Check sheet for the modelled part. Datum: model origin and axes. Units: mm. Face numbers are marked on the shaded views. Give positions to 0.01 mm unless a question says otherwise; leave off trailing zeros. Write each loop counter-clockwise with the first axis right and the second up, starting at its lowest first coordinate (ties: lowest second). Pieces come first, ordered by that corner, then holes. Notation, with made-up numbers: M 2.25,26.25 L 57.25,26.25 A15 cw 57.25,38.25 Z; hole C 89,89 d2. An arc over 180 degrees is marked long. Use CSV: the item, a comma, the result in double quotes. Start each with the question number.
1. Scan lines: line 1 (Y direction, x = 0, z = 7); line 2 (Z direction, x = 18.5, y = 7); line 3 (Z direction, x = 4, y = -2). Record each from-to range of solid material in increasing order.
2. Cross-section at B-B, the plane y = 38.5. Enter the section's corners in (x, z).
3. Mould release check, pull along X, two halves, no side actions. Record for the marked faces 1, 2 and 3: +X half, -X half, draft (parallel to the pull), parting line (faces both ways), or undercut.
4. Cross-section at C-C, the plane z = 6.5. Enter the section's corners in (x, y), and give its area (3 significant figures).
5. Depth check by flat-ended pin: P1, Ø3, axis at y = -1, z = 20.5, coming from the +X side; P2, Ø8, axis at x = -7, y = 43.5, coming from the -Z side; P3, Ø10, axis at x = -52, z = 5, coming from the +Y side; P4, Ø2, axis at x = 9.5, z = 28, coming from the -Y side. Enter the tip coordinate at first touch or a pass-through.
6. Cross-section at A-A, the plane x = 52. Enter the section's corners in (y, z).
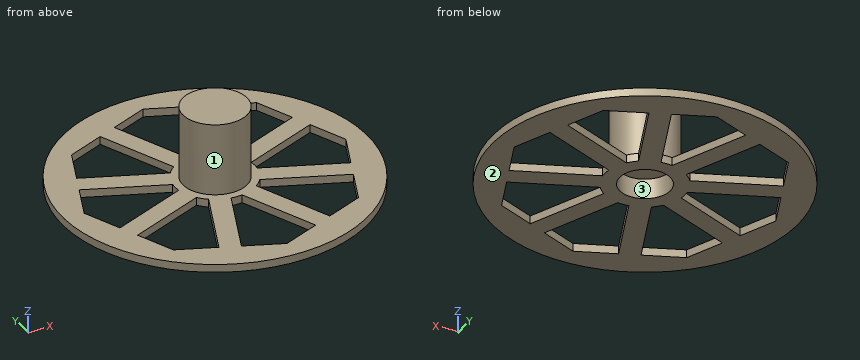
from build123d import *

# Parameters (mm, degrees)
F0_R     = 16
F1_DEPTH = 40
F2_R     = 12.6
F3_DEPTH = 10
F4_R     = 76
F4_R_2   = 16
F5_DEPTH = 4
F7_DEPTH = 4


with BuildPart() as f1:
    # F0 (on Top) → F1 (new body)
    with BuildSketch(Plane.XY):
        Circle(F0_R)
    extrude(amount=F1_DEPTH)

    # F2 (on face) → F3 (cut)
    with BuildSketch(Plane(origin=(0, 0, 0), x_dir=(1, 0, 0), z_dir=(0, 0, -1))):
        Circle(F2_R)
    extrude(amount=-F3_DEPTH, mode=Mode.SUBTRACT)

    # F4 (on Top) → F5 (join)
    with BuildSketch(Plane.XY):
        Circle(F4_R)
        Circle(F4_R_2, mode=Mode.SUBTRACT)
    extrude(amount=F5_DEPTH)

    # F6 (on face) → F7 (cut, through all)
    with BuildSketch(Plane.XY.offset(4)):
        with BuildLine():
            Line((27.953921, -54.421107), (46.669048, -46.669048))
            Line((46.669048, -46.669048), (54.421107, -27.953921))
            Line((54.421107, -27.953921), (15.977433, -12.03003))
            ThreePointArc((15.977433, -12.03003), (14.142136, -14.142136), (12.03003, -15.977433))
            Line((12.03003, -15.977433), (27.953921, -54.421107))
        make_face()
        with BuildLine():
            Line((-18.715126, -58.247941), (0, -66))
            Line((0, -66), (18.715126, -58.247941))
            Line((18.715126, -58.247941), (2.791235, -19.804267))
            ThreePointArc((2.791235, -19.804267), (0, -20), (-2.791235, -19.804267))
            Line((-2.791235, -19.804267), (-18.715126, -58.247941))
        make_face()
        with BuildLine():
            Line((-54.421107, -27.953921), (-46.669048, -46.669048))
            Line((-46.669048, -46.669048), (-27.953921, -54.421107))
            Line((-27.953921, -54.421107), (-12.03003, -15.977433))
            ThreePointArc((-12.03003, -15.977433), (-14.142136, -14.142136), (-15.977433, -12.03003))
            Line((-15.977433, -12.03003), (-54.421107, -27.953921))
        make_face()
        with BuildLine():
            Line((-58.247941, 18.715126), (-66, 0))
            Line((-66, 0), (-58.247941, -18.715126))
            Line((-58.247941, -18.715126), (-19.804267, -2.791235))
            ThreePointArc((-19.804267, -2.791235), (-20, 0), (-19.804267, 2.791235))
            Line((-19.804267, 2.791235), (-58.247941, 18.715126))
        make_face()
        with BuildLine():
            Line((-27.953921, 54.421107), (-46.669048, 46.669048))
            Line((-46.669048, 46.669048), (-54.421107, 27.953921))
            Line((-54.421107, 27.953921), (-15.977433, 12.03003))
            ThreePointArc((-15.977433, 12.03003), (-14.142136, 14.142136), (-12.03003, 15.977433))
            Line((-12.03003, 15.977433), (-27.953921, 54.421107))
        make_face()
        with BuildLine():
            Line((18.715126, 58.247941), (0, 66))
            Line((0, 66), (-18.715126, 58.247941))
            Line((-18.715126, 58.247941), (-2.791235, 19.804267))
            ThreePointArc((-2.791235, 19.804267), (0, 20), (2.791235, 19.804267))
            Line((2.791235, 19.804267), (18.715126, 58.247941))
        make_face()
        with BuildLine():
            Line((54.421107, 27.953921), (46.669048, 46.669048))
            Line((46.669048, 46.669048), (27.953921, 54.421107))
            Line((27.953921, 54.421107), (12.03003, 15.977433))
            ThreePointArc((12.03003, 15.977433), (14.142136, 14.142136), (15.977433, 12.03003))
            Line((15.977433, 12.03003), (54.421107, 27.953921))
        make_face()
        with BuildLine():
            Line((58.247941, -18.715126), (66, 0))
            Line((66, 0), (58.247941, 18.715126))
            Line((58.247941, 18.715126), (19.804267, 2.791235))
            ThreePointArc((19.804267, 2.791235), (20, 0), (19.804267, -2.791235))
            Line((19.804267, -2.791235), (58.247941, -18.715126))
        make_face()
    extrude(amount=-F7_DEPTH, mode=Mode.SUBTRACT)


solid = f1.part
Worked answers:
1,line 1,"y = -16 to -12.6, 12.6 to 16"
1,line 2,"z = 0 to 4"
1,line 3,"z = 10 to 40"
2,outline,"M -65.53,0 L -50.05,0 L -50.05,4 L -65.53,4 Z; M -21.36,0 L -10.54,0 L -10.54,4 L -21.36,4 Z; M 10.54,0 L 21.36,0 L 21.36,4 L 10.54,4 Z; M 50.05,0 L 65.53,0 L 65.53,4 L 50.05,4 Z"
3,face 1,"parting line"
3,face 2,"draft"
3,face 3,"undercut"
4,outline,"C 0,0 d32; hole C 0,0 d25.2"
4,area,"305 mm^2"
5,P1,"stops at x = 16"
5,P2,"passes through"
5,P3,"stops at y = 59.64"
5,P4,"stops at y = -13.56"
6,outline,"M -55.43,0 L -33.8,0 L -33.8,4 L -55.43,4 Z; M -26.95,0 L -16.13,0 L -16.13,4 L -26.95,4 Z; M 16.13,0 L 26.95,0 L 26.95,4 L 16.13,4 Z; M 33.8,0 L 55.43,0 L 55.43,4 L 33.8,4 Z"
